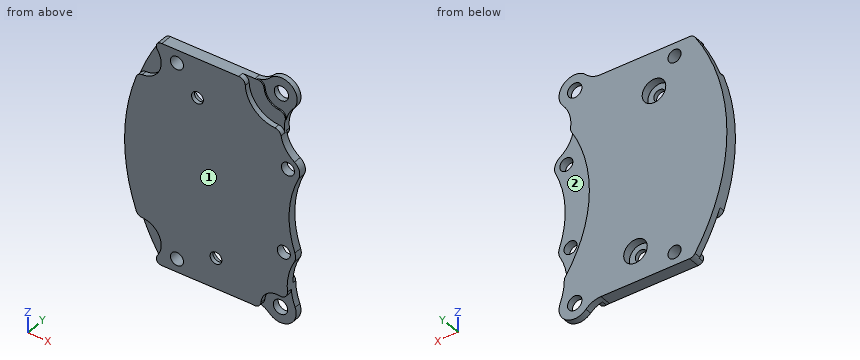
from build123d import *

# Parameters (mm, degrees)
SKETCH_1_R          = 0.5
SKETCH_1_R_2        = 0.55
SKETCH_1_R_3        = 0.45
EXTRUDE_1_DEPTH     = 0.9
SKETCH_2_R          = 10.1
CUT_EXTRUDE_1_DEPTH = 0.3
SKETCH_3_R          = 2.4
SKETCH_3_R_2        = 1.5
CUT_EXTRUDE_2_DEPTH = 0.4
SKETCH_4_R          = 1.25
CUT_EXTRUDE_3_DEPTH = 0.1
SKETCH_5_R          = 0.9
CUT_EXTRUDE_4_DEPTH = 0.6
SKETCH_6_R          = 1.2
CUT_EXTRUDE_5_DEPTH = 0.4
FILLET_START        = -1
FILLET_1_DEPTH      = 1.4
FILLET_START_2      = 0.4
FILLET_1_2_DEPTH    = 0.1
FILLET_START_3      = 0.5
FILLET_1_3_DEPTH    = 1.5
FILLET_START_4      = 0.6
FILLET_1_4_DEPTH    = 1.4


with BuildPart() as part:
    # Эскиз1 → Бобышка-Вытянуть1 (new body)
    with BuildSketch(Plane(origin=(0, 0, 0), x_dir=(1, 0, 0), z_dir=(0, 1, 0))):
        with BuildLine():
            Line((-8.874701271, 0), (-1.795461863, 0))
            ThreePointArc((-1.795461863, 0), (-1.203537037, -0.121731158), (-0.70768647, -0.467166667))
            ThreePointArc((-0.70768647, -0.467166667), (0.973552797, -0.525347996), (1.060942394, 1.154626289))
            ThreePointArc((1.060942394, 1.154626289), (0.477391661, 3.052026669), (1.522351258, 4.739841558))
            ThreePointArc((1.522351258, 4.739841558), (1.889015496, 5.247769663), (1.835416111, 5.871917665))
            ThreePointArc((1.835416111, 5.871917665), (1.116849218, 8.747445681), (1.55283729, 11.679154083))
            ThreePointArc((1.55283729, 11.679154083), (1.603016133, 12.049823116), (1.498169999, 12.408878456))
            ThreePointArc((1.498169999, 12.408878456), (0.968934134, 14.279432184), (1.278077174, 16.198674855))
            ThreePointArc((1.278077174, 16.198674855), (0.816325951, 17.647158357), (-0.694815473, 17.480514286))
            ThreePointArc((-0.694815473, 17.480514286), (-1.217938679, 17.125012349), (-1.837947895, 17))
            Line((-1.837947895, 17), (-8.874701271, 17))
            ThreePointArc((-8.874701271, 17), (-11.453066156, 8.5), (-8.874701271, 0))
        make_face()
        with Locations(Location((1.021573168, 5.487652568, 0), (0, 0, 270))):
            Circle(SKETCH_1_R, mode=Mode.SUBTRACT)
        with Locations(Location((0.162533844, 0.3591, 0), (0, 0, 270))):
            Circle(SKETCH_1_R_2, mode=Mode.SUBTRACT)
        with Locations(Location((-5.887426867, 2.992111817, 0), (0, 0, 270))):
            Circle(SKETCH_1_R_3, mode=Mode.SUBTRACT)
        with Locations(Location((-7.453066156, 1, 0), (0, 0, 270))):
            Circle(SKETCH_1_R, mode=Mode.SUBTRACT)
        with Locations(Location((-4.474879967, 14.65491132, 0), (0, 0, 270))):
            Circle(SKETCH_1_R_3, mode=Mode.SUBTRACT)
        with Locations(Location((-7.453066156, 16, 0), (0, 0, 90))):
            Circle(SKETCH_1_R, mode=Mode.SUBTRACT)
        with Locations(Location((0.705531067, 11.982588035, 0), (0, 0, 270))):
            Circle(SKETCH_1_R, mode=Mode.SUBTRACT)
        with Locations(Location((0.162533844, 16.6409, 0), (0, 0, 270))):
            Circle(SKETCH_1_R_2, mode=Mode.SUBTRACT)
    extrude(amount=EXTRUDE_1_DEPTH)

    # Эскиз2 → Вырез-Вытянуть1 (cut)
    with BuildSketch(Plane(origin=(0, 0.9, 0), x_dir=(1, 0, 0), z_dir=(0, 1, 0))):
        with Locations((9.146933844, 8.5)):
            Circle(SKETCH_2_R)
    extrude(amount=-CUT_EXTRUDE_1_DEPTH, mode=Mode.SUBTRACT)

    # Эскиз3 → Вырез-Вытянуть2 (cut)
    with BuildSketch(Plane.XZ):
        with Locations((0.162533844, -0.3591)):
            Circle(SKETCH_3_R)
        with Locations((-10.155327835, -1.531617514)):
            Circle(SKETCH_3_R_2)
        with Locations((-10.155327835, -15.468382486)):
            Circle(SKETCH_3_R_2)
    extrude(amount=-CUT_EXTRUDE_2_DEPTH, mode=Mode.SUBTRACT)

    # Эскиз4 → Вырез-Вытянуть3 (cut)
    with BuildSketch(Plane.XZ.offset(-0.4)):
        with Locations((0.162533844, -0.3591)):
            Circle(SKETCH_4_R)
    extrude(amount=-CUT_EXTRUDE_3_DEPTH, mode=Mode.SUBTRACT)

    # Эскиз5 → Вырез-Вытянуть4 (cut)
    with BuildSketch(Plane(origin=(0, 0.9, 0), x_dir=(1, 0, 0), z_dir=(0, 1, 0))):
        with Locations(Location((-5.887426867, 2.992111817, 0), (0, 0, 270))):
            Circle(SKETCH_5_R)
        with Locations(Location((-4.474879967, 14.65491132, 0), (0, 0, 270))):
            Circle(SKETCH_5_R)
    extrude(amount=-CUT_EXTRUDE_4_DEPTH, mode=Mode.SUBTRACT)

    # Эскиз6 → Вырез-Вытянуть5 (cut)
    with BuildSketch(Plane.XZ):
        with Locations((0.162533844, -16.6409)):
            Circle(SKETCH_6_R)
    extrude(amount=-CUT_EXTRUDE_5_DEPTH, mode=Mode.SUBTRACT)

    # Скругление1: read off the stored shape, not the designer's step
    # Скругление1 outline → Скругление1 (cut)
    with BuildSketch(Plane(origin=(0, 0, 0), x_dir=(1, 0, 0), z_dir=(0, 1, 0)).offset(FILLET_START)):
        with BuildLine():
            ThreePointArc((-10.564834765, 13.6372099), (-10.388255808, 13.873471068), (-10.10922841, 13.969091039))
            ThreePointArc((-10.10922841, 13.969091039), (-10.271568069, 13.972893199), (-10.432545463, 13.994221577))
            ThreePointArc((-10.432545463, 13.994221577), (-10.499800665, 13.816127249), (-10.564834765, 13.6372099))
        make_face()
        with BuildLine():
            ThreePointArc((-9.146480388, 16.578439614), (-9.032397619, 16.462881218), (-8.931474904, 16.335667907))
            ThreePointArc((-8.931474904, 16.335667907), (-9.021275661, 16.577400508), (-8.978676793, 16.831731322))
            ThreePointArc((-8.978676793, 16.831731322), (-8.809674916, 16.955996525), (-8.604572089, 17))
            Line((-8.604572089, 17), (-8.874701271, 17))
            ThreePointArc((-8.874701271, 17), (-8.950481675, 16.885472917), (-9.025231073, 16.77027027))
            ThreePointArc((-9.025231073, 16.77027027), (-9.086211401, 16.674579749), (-9.146480388, 16.578439614))
        make_face()
        with BuildLine():
            ThreePointArc((-10.10922841, 3.030908961), (-10.388255808, 3.126528932), (-10.564834765, 3.3627901))
            ThreePointArc((-10.564834765, 3.3627901), (-10.499800665, 3.183872751), (-10.432545462, 3.005778423))
            ThreePointArc((-10.432545462, 3.005778423), (-10.271568069, 3.027106801), (-10.10922841, 3.030908961))
        make_face()
        with BuildLine():
            ThreePointArc((-8.978676793, 0.168268678), (-9.021275661, 0.422599492), (-8.931474903, 0.664332093))
            ThreePointArc((-8.931474903, 0.664332093), (-9.032397619, 0.537118782), (-9.146480388, 0.421560386))
            ThreePointArc((-9.146480388, 0.421560386), (-9.086211401, 0.325420251), (-9.025231073, 0.22972973))
            ThreePointArc((-9.025231073, 0.22972973), (-8.950481675, 0.114527083), (-8.874701271, 0))
            Line((-8.874701271, 0), (-8.604572089, 0))
            ThreePointArc((-8.604572089, 0), (-8.809674916, 0.044003475), (-8.978676793, 0.168268678))
        make_face()
        with BuildLine():
            ThreePointArc((-0.694815473, 17.480514286), (-1.112314109, 17.17400715), (-1.605848887, 17.016923865))
            ThreePointArc((-1.605848887, 17.016923865), (-1.219826633, 16.911729191), (-1.034538008, 16.557120639))
            ThreePointArc((-1.034538008, 16.557120639), (-0.963665757, 17.055236166), (-0.694815473, 17.480514286))
        make_face()
        with BuildLine():
            ThreePointArc((-2.234631739, 0.475706897), (-2.389183693, 0.137959566), (-2.734041235, 0))
            Line((-2.734041235, 0), (-2.210448918, 0))
            ThreePointArc((-2.210448918, 0), (-2.23437105, 0.237252027), (-2.234631739, 0.475706897))
        make_face()
        with BuildLine():
            ThreePointArc((1.278077174, 16.198674855), (0.926926141, 15.715857074), (0.386577368, 15.462000301))
            ThreePointArc((0.386577368, 15.462000301), (0.815072231, 15.341843176), (0.978072419, 14.92774594))
            ThreePointArc((0.978072419, 14.92774594), (1.081728132, 15.5741506), (1.278077174, 16.198674855))
        make_face()
        with BuildLine():
            ThreePointArc((0.030324762, 2.755455725), (0.244370036, 2.757704352), (0.457764308, 2.740872234))
            ThreePointArc((0.457764308, 2.740872234), (0.466881934, 2.954735051), (0.495018839, 3.16693484))
            ThreePointArc((0.495018839, 3.16693484), (0.33425049, 2.880359605), (0.030324762, 2.755455725))
        make_face()
    extrude(amount=FILLET_1_DEPTH, mode=Mode.SUBTRACT)

    # Fillet 1 2 outline → Fillet 1 2 (cut)
    with BuildSketch(Plane(origin=(0, 0, 0), x_dir=(1, 0, 0), z_dir=(0, 1, 0)).offset(FILLET_START_2)):
        with BuildLine():
            ThreePointArc((-9.025231073, 16.77027027), (-8.844222736, 16.938825213), (-8.604572089, 17))
            Line((-8.604572089, 17), (-8.874701271, 17))
            ThreePointArc((-8.874701271, 17), (-8.950481675, 16.885472917), (-9.025231073, 16.77027027))
        make_face()
        with BuildLine():
            ThreePointArc((-8.604572089, 0), (-8.844222736, 0.061174787), (-9.025231073, 0.22972973))
            ThreePointArc((-9.025231073, 0.22972973), (-8.950481675, 0.114527083), (-8.874701271, 0))
            Line((-8.874701271, 0), (-8.604572089, 0))
        make_face()
        with BuildLine():
            ThreePointArc((-1.08403646, 0.451633648), (-1.262452429, 0.10463646), (-1.635863903, -0.00851467))
            ThreePointArc((-1.635863903, -0.00851467), (-1.25040696, -0.102532593), (-0.903083615, -0.294321327))
            ThreePointArc((-0.903083615, -0.294321327), (-1.052235792, 0.064422668), (-1.08403646, 0.451633648))
        make_face()
        with BuildLine():
            ThreePointArc((0.884565826, 1.379477291), (0.660848396, 1.77945859), (0.517239852, 2.214672463))
            ThreePointArc((0.517239852, 2.214672463), (0.431918135, 1.807119305), (0.067603665, 1.605490092))
            ThreePointArc((0.067603665, 1.605490092), (0.49582743, 1.563847021), (0.884565826, 1.379477291))
        make_face()
    extrude(amount=FILLET_1_2_DEPTH, mode=Mode.SUBTRACT)

    # Fillet 1 3 outline → Fillet 1 3 (cut)
    with BuildSketch(Plane(origin=(0, 0, 0), x_dir=(1, 0, 0), z_dir=(0, 1, 0)).offset(FILLET_START_3)):
        with BuildLine():
            ThreePointArc((-9.025231073, 16.77027027), (-8.844222736, 16.938825213), (-8.604572089, 17))
            Line((-8.604572089, 17), (-8.874701271, 17))
            ThreePointArc((-8.874701271, 17), (-8.950481675, 16.885472917), (-9.025231073, 16.77027027))
        make_face()
        with BuildLine():
            ThreePointArc((-8.604572089, 0), (-8.844222736, 0.061174787), (-9.025231073, 0.22972973))
            ThreePointArc((-9.025231073, 0.22972973), (-8.950481675, 0.114527083), (-8.874701271, 0))
            Line((-8.874701271, 0), (-8.604572089, 0))
        make_face()
    extrude(amount=FILLET_1_3_DEPTH, mode=Mode.SUBTRACT)

    # Fillet 1 4 outline → Fillet 1 4 (cut)
    with BuildSketch(Plane(origin=(0, 0, 0), x_dir=(1, 0, 0), z_dir=(0, 1, 0)).offset(FILLET_START_4)):
        with BuildLine():
            ThreePointArc((0.963003545, 14.4188922), (0.96158445, 14.49585524), (0.961482029, 14.572831294))
            ThreePointArc((0.961482029, 14.572831294), (0.937837832, 14.424463631), (0.871185578, 14.289817841))
            ThreePointArc((0.871185578, 14.289817841), (0.916841519, 14.354535024), (0.963003545, 14.4188922))
        make_face()
        with BuildLine():
            ThreePointArc((0.42008242, 3.415507477), (0.478926522, 3.25893209), (0.482835834, 3.091710089))
            ThreePointArc((0.482835834, 3.091710089), (0.496570271, 3.175545649), (0.513263178, 3.258842605))
            ThreePointArc((0.513263178, 3.258842605), (0.466319363, 3.336964825), (0.42008242, 3.415507477))
        make_face()
    extrude(amount=FILLET_1_4_DEPTH, mode=Mode.SUBTRACT)


solid = part.part
Could you check a few things on this model? Use its own coordinates, in mm. Face numbers are marked on the shaded views. Round coordinates to 2 decimals unless told otherwise and drop trailing zeros. Write each loop counter-clockwise with the first axis right and the second up, starting at its lowest first coordinate (ties: lowest second). Pieces come first, ordered by that corner, then holes. Notation, with made-up numbers: (71, 23) -> (115, 23) arc R21 cw to (115, 46) -> close; hole circle Ø11 at (20.25, 17). An arc over 180 degrees is marked (long way). Use a Markdown table: item, result.
1. If we section it at C-C (z = -8): List the corners of the cut face in (x, y) for me.
Answer key:
| item | result |
|---|---|
| outline | (-11.44, 0) -> (1.19, 0) -> (1.19, 0.6) -> (-0.94, 0.6) -> (-0.94, 0.9) -> (-11.44, 0.9) -> close |
2. For pin 1 Ø3 at (x, z) = (0.5, -7.5) entering from +Y; pin 2 Ø1.4 at (x, z) = (0.16, -16.64) entering from -Y; pin 3 Ø0.5 at (x, z) = (-4.5, -15) entering from +Y, each with a flat end and sliding along its axis, tell me the tip position at first contact or that it passes through.
Answer key:
| item | result |
|---|---|
| pin 1 | stops at y = 0.9 |
| pin 2 | stops at y = 0.4 |
| pin 3 | stops at y = 0.3 |
3. We'd pull the mould along Z, two halves only. Please class the marked faces 1 and 2: +Z half, -Z half, draft (parallel to the pull), parting line (faces both ways), or undercut.
Answer key:
| item | result |
|---|---|
| face 1 | draft |
| face 2 | undercut |
4. If we section it at A-A (z = -5.25): List the corners of the cut face in (x, y) for me.
Answer key:
| item | result |
|---|---|
| outline | (-11.1, 0) -> (0.58, 0) -> (0.58, 0.6) -> (-0.42, 0.6) -> (-0.42, 0.9) -> (-11.1, 0.9) -> close; (1.46, 0) -> (1.89, 0) -> (1.89, 0.6) -> (1.46, 0.6) -> close |
5. Please list where these lines run through material, in increasing order: probe 1 along Z at (x, y) = (-8.5, 0.45); probe 2 along Z at (x, y) = (-6.25, 0.5); probe 3 along X at (y, z) = (0.75, -1.25).
Answer key:
| item | result |
|---|---|
| probe 1 | z = -17 to 0 |
| probe 2 | z = -17 to -3.82, -2.17 to 0 |
| probe 3 | x = -9.63 to -7.89, -7.02 to 0.98 |
6. If we section it at B-B (z = -10.25): List the corners of the cut face in (x, y) for me.
Answer key:
| item | result |
|---|---|
| outline | (-11.35, 0) -> (1.19, 0) -> (1.19, 0.6) -> (-0.8, 0.6) -> (-0.8, 0.9) -> (-11.35, 0.9) -> close |
